Design review of the part built by this model. Coordinates are the model's own, in mm. Coordinates: 2 decimals unless noted, no trailing zeros. Loops run counter-clockwise (first coordinate to the right, second up) from the corner with the lowest first, then second, coordinate; pieces in that order, holes last. Notation, with made-up numbers: M 19.5,79 L 57.5,79 A16 ccw 57.5,107 Z; hole C 30.5,64.5 d11. An arc over 180 degrees is marked long. Put each result on its own line as item: value. Start each with the question number.
(1) Clearance check with flat-ended pins moving along their axes: pin 1 (0.6 mm diameter, centred on y = -38.5, z = 1, fed in from -X); pin 2 (1 mm diameter, centred on x = 22.5, z = 0.5, fed in from +Y); pin 3 (0.6 mm diameter, centred on x = 47, z = 1, fed in from -Y); pin 4 (9.5 mm diameter, centred on x = 14.67, y = 38.64, fed in from +Z). State where each tip first meets the part, or that it passes through.
(2) Take a section at A-A, the plane x = 52. Give the boundary of the cut face in (y, z).
(3) Take a section at C-C, the plane x = 4.5. Give the boundary of the cut face in (y, z), then the cut area to 3 significant figures.
(4) Take a section at D-D, the plane z = 1.35. Count the separate pieces of the cut face and the enclosed holes in it, then the cut area to 3 significant figures.
(5) For probe 1 along Y at (x, z) = (0, 1.3); probe 2 along X at (y, z) = (-39, 0.4); probe 3 along X at (y, z) = (38.5, 0.3), list the stretches that pass through material, from the lowest coordinate up. Write a range as [from, to].
(6) Take a section at B-B, the plane x = -20. Give the boundary of the cut face in (y, z), then the cut area to 3 significant figures.
```python
from build123d import *

# Parameters (mm, degrees)
SKETCH_1_R      = 2
SKETCH_1_R_2    = 1.5
SKETCH_1_R_3    = 6.5
SKETCH_1_R_4    = 0.75
SKETCH_1_R_5    = 6
EXTRUDE_1_DEPTH = 2


with BuildPart() as part:
    # 草图1 → 凸台-拉伸1 (new body)
    with BuildSketch(Plane.XY):
        with BuildLine():
            Line((58.445187997, 32.9), (74.5685, 32.9))
            ThreePointArc((74.5685, 32.9), (75.982713562, 32.314213562), (76.5685, 30.9))
            Line((76.5685, 30.9), (76.5685, -30.9))
            ThreePointArc((76.5685, -30.9), (75.982713562, -32.314213562), (74.5685, -32.9))
            Line((74.5685, -32.9), (58.445187997, -32.9))
            ThreePointArc((58.445187997, -32.9), (53.927025417, -33.978889817), (50.383782756, -36.982758621))
            ThreePointArc((50.383782756, -36.982758621), (-62.5, 0), (50.383782756, 36.982758621))
            ThreePointArc((50.383782756, 36.982758621), (53.927025417, 33.978889817), (58.445187997, 32.9))
        make_face()
        with Locations((0, -20)):
            Circle(SKETCH_1_R, mode=Mode.SUBTRACT)
        with Locations((0, -59)):
            Circle(SKETCH_1_R_2, mode=Mode.SUBTRACT)
        with Locations((-20, 0)):
            Circle(SKETCH_1_R, mode=Mode.SUBTRACT)
        with Locations((0, 20)):
            Circle(SKETCH_1_R, mode=Mode.SUBTRACT)
        with Locations((20, 0)):
            Circle(SKETCH_1_R, mode=Mode.SUBTRACT)
        with Locations((-31.89780823, -49.633958437)):
            Circle(SKETCH_1_R_2, mode=Mode.SUBTRACT)
        with Locations((-53.668287726, -24.509485767)):
            Circle(SKETCH_1_R_2, mode=Mode.SUBTRACT)
        with Locations((-58.399465071, 8.396575458)):
            Circle(SKETCH_1_R_2, mode=Mode.SUBTRACT)
        with Locations((-44.589224887, 38.636783303)):
            Circle(SKETCH_1_R_2, mode=Mode.SUBTRACT)
        with Locations((-16.622220854, 56.610085443)):
            Circle(SKETCH_1_R_2, mode=Mode.SUBTRACT)
        with Locations((16.622220854, 56.610085443)):
            Circle(SKETCH_1_R_2, mode=Mode.SUBTRACT)
        with Locations((44.589224887, 38.636783303)):
            Circle(SKETCH_1_R_2, mode=Mode.SUBTRACT)
        with Locations((31.89780823, -49.633958437)):
            Circle(SKETCH_1_R_2, mode=Mode.SUBTRACT)
        Circle(SKETCH_1_R_3, mode=Mode.SUBTRACT)
        with Locations((-7.498513861, -7.498513861)):
            Circle(SKETCH_1_R_4, mode=Mode.SUBTRACT)
        with Locations((-7.498513861, 7.498513861)):
            Circle(SKETCH_1_R_4, mode=Mode.SUBTRACT)
        with Locations((7.498513861, 7.498513861)):
            Circle(SKETCH_1_R_4, mode=Mode.SUBTRACT)
        with Locations((7.498513861, -7.498513861)):
            Circle(SKETCH_1_R_4, mode=Mode.SUBTRACT)
        with Locations((14.6685, 38.636783303)):
            Circle(SKETCH_1_R_5, mode=Mode.SUBTRACT)
        with Locations(Location((14.6685, -38.636783303, 0), (0, 0, 180))):
            Circle(SKETCH_1_R_5, mode=Mode.SUBTRACT)
        with BuildLine():
            Line((-46.475800154, 4), (-27.110883423, 4))
            ThreePointArc((-27.110883423, 4), (-25.273766116, 4.628291755), (-24.206145914, 6.25))
            ThreePointArc((-24.206145914, 6.25), (-17.67766953, 17.67766953), (-6.25, 24.206145914))
            ThreePointArc((-6.25, 24.206145914), (-4.628291755, 25.273766116), (-4, 27.110883423))
            Line((-4, 27.110883423), (-4, 46.475800154))
            ThreePointArc((-4, 46.475800154), (-5.043015781, 48.749610341), (-7.446808511, 49.44234059))
            ThreePointArc((-7.446808511, 49.44234059), (-35.355339059, 35.355339059), (-49.44234059, 7.446808511))
            ThreePointArc((-49.44234059, 7.446808511), (-48.749610341, 5.043015781), (-46.475800154, 4))
        make_face(mode=Mode.SUBTRACT)
        with BuildLine():
            Line((-27.110883423, -4), (-46.475800154, -4))
            ThreePointArc((-46.475800154, -4), (-48.749610341, -5.043015781), (-49.44234059, -7.446808511))
            ThreePointArc((-49.44234059, -7.446808511), (-35.355339059, -35.355339059), (-7.446808511, -49.44234059))
            ThreePointArc((-7.446808511, -49.44234059), (-5.043015781, -48.749610341), (-4, -46.475800154))
            Line((-4, -46.475800154), (-4, -27.110883423))
            ThreePointArc((-4, -27.110883423), (-4.628291755, -25.273766116), (-6.25, -24.206145914))
            ThreePointArc((-6.25, -24.206145914), (-17.67766953, -17.67766953), (-24.206145914, -6.25))
            ThreePointArc((-24.206145914, -6.25), (-25.273766116, -4.628291755), (-27.110883423, -4))
        make_face(mode=Mode.SUBTRACT)
        with BuildLine():
            Line((20.6685, -24.4), (26.6685, -24.4))
            ThreePointArc((26.6685, -24.4), (28.1685, -25.9), (26.6685, -27.4))
            Line((26.6685, -27.4), (20.6685, -27.4))
            ThreePointArc((20.6685, -27.4), (19.1685, -25.9), (20.6685, -24.4))
        make_face(mode=Mode.SUBTRACT)
        with BuildLine():
            Line((20.6685, 27.4), (26.6685, 27.4))
            ThreePointArc((26.6685, 27.4), (28.1685, 25.9), (26.6685, 24.4))
            Line((26.6685, 24.4), (20.6685, 24.4))
            ThreePointArc((20.6685, 24.4), (19.1685, 25.9), (20.6685, 27.4))
        make_face(mode=Mode.SUBTRACT)
        with BuildLine():
            Line((64.5685, 27.4), (70.5685, 27.4))
            ThreePointArc((70.5685, 27.4), (72.0685, 25.9), (70.5685, 24.4))
            Line((70.5685, 24.4), (64.5685, 24.4))
            ThreePointArc((64.5685, 24.4), (63.0685, 25.9), (64.5685, 27.4))
        make_face(mode=Mode.SUBTRACT)
        with BuildLine():
            Line((64.5685, -24.4), (70.5685, -24.4))
            ThreePointArc((70.5685, -24.4), (72.0685, -25.9), (70.5685, -27.4))
            Line((70.5685, -27.4), (64.5685, -27.4))
            ThreePointArc((64.5685, -27.4), (63.0685, -25.9), (64.5685, -24.4))
        make_face(mode=Mode.SUBTRACT)
        with BuildLine():
            Line((27.6685, 20.9), (57.5685, 20.9))
            ThreePointArc((57.5685, 20.9), (58.982713562, 20.314213562), (59.5685, 18.9))
            Line((59.5685, 18.9), (59.5685, -18.9))
            ThreePointArc((59.5685, -18.9), (58.982713562, -20.314213562), (57.5685, -20.9))
            Line((57.5685, -20.9), (27.6685, -20.9))
            ThreePointArc((27.6685, -20.9), (26.254286438, -20.314213562), (25.6685, -18.9))
            Line((25.6685, -18.9), (25.6685, 18.9))
            ThreePointArc((25.6685, 18.9), (26.254286438, 20.314213562), (27.6685, 20.9))
        make_face(mode=Mode.SUBTRACT)
    extrude(amount=EXTRUDE_1_DEPTH)


solid = part.part
```
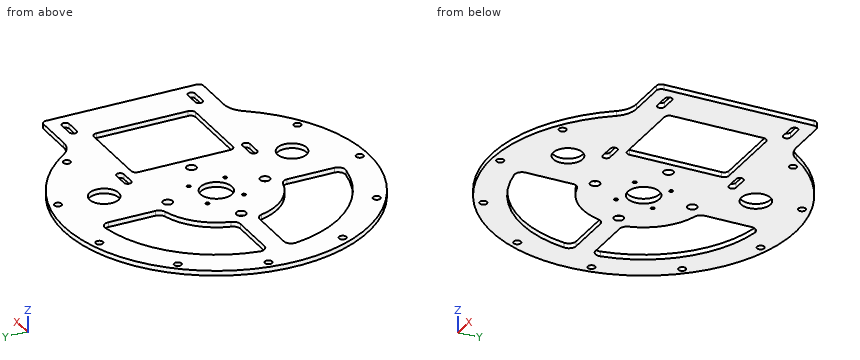
Computed values:
1. pin 1: stops at x = -49.47
1. pin 2: stops at y = 58.5
1. pin 3: stops at y = -41.54
1. pin 4: passes through
2. outline: M -35.25,0 L -20.9,0 L -20.9,2 L -35.25,2 Z; M 20.9,0 L 35.25,0 L 35.25,2 L 20.9,2 Z
3. outline: M -62.34,0 L -4.69,0 L -4.69,2 L -62.34,2 Z; M 4.69,0 L 62.34,0 L 62.34,2 L 4.69,2 Z
3. area: 231 mm^2
4. separate pieces: 1
4. enclosed holes: 27
4. area: 8,880 mm^2
5. probe 1: y = [-62.5, -60.5], [-57.5, -22], [-18, -6.5], [6.5, 18], [22, 62.5]
5. probe 2: x = [-48.84, -31.29], [-4, 8.68], [20.66, 48.84]
5. probe 3: x = [-49.23, -46.08], [-43.1, -31.9], [-4, 8.67], [20.67, 43.1], [46.08, 49.23]
6. outline: M -59.21,0 L -45.83,0 L -45.83,2 L -59.21,2 Z; M -15,0 L -2,0 L -2,2 L -15,2 Z; M 2,0 L 15,0 L 15,2 L 2,2 Z; M 45.83,0 L 59.21,0 L 59.21,2 L 45.83,2 Z
6. area: 106 mm^2
